Geometry: final body of the model. Coordinates: model frame, mm. Round coordinates to 2 decimals unless told otherwise and drop trailing zeros. Order: outer loops, then holes, each group sorted by start corner. A loop starts at its lowest first (then second) coordinate and runs counter-clockwise, first axis right, second up. Notation, with made-up numbers: M -11,-26 L 8,-26 A21 ccw 8,10 Z; hole C 57,-18 d8. An arc over 180 degrees is marked long. Return JSON: item names as keys, results as strings. Group by question number.
Q1. Ray query, probe 1 along X at (y, z) = (0, -0.6); probe 2 along Y at (x, z) = (1.75, -0.45); probe 3 along Y at (x, z) = (-1, -1.3). Return the intervals inside material, ascending.
Q2. Cut plane C-C on z = -0.8. Output: boundary loops of the cut face in (x, y).
Q3. Cut plane B-B on y = 0. Output: boundary loops of the cut face in (x, z).
Q4. Cut plane A-A on x = 0. Output: boundary loops of the cut face in (y, z).
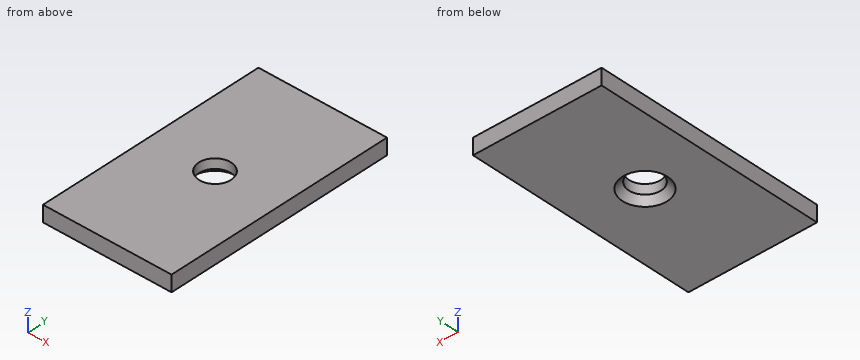
Autodesk Inventor part; units mm, degrees
ref_plane "to_magnet_XY" through (0, 0, 0) normal (0, 0, 1) x (1, 0, 0)
ref_plane "to_magnet_YZ" through (0, 0, 0) normal (1, 0, 0) x (0, 1, 0)
ref_plane "to_magnet_ZX" through (0, 0, 0) normal (0, 1, 0) x (0, 0, 1)
sketch "Sketch_1" plane through (0, 0, 0) normal (0, 0, 1) x (1, 0, 0)
  line L0 (-8, 14.5) -> (-8, -14.5)
  line L1 (-8, -14.5) -> (8, -14.5)
  line L2 (8, -14.5) -> (8, 14.5)
  line L3 (8, 14.5) -> (-8, 14.5)
extrude "Extrusion1" add sketch "Sketch_1" against normal blind 2
sketch "Sketch_2" plane through (0, 0, 0) normal (1, 0, 0) x (0, 1, 0)
  line L0 (0, -2) -> (0, 0)
  line L1 (0, 0) -> (2, 0)
  line L2 (2, 0) -> (2, -1.2)
  line L3 (2, -1.2) -> (2.8, -2)
  line L4 (2.8, -2) -> (0, -2)
  line L5 (0, -2) -> (0, 0)
revolve "Revolution1" cut sketch "Sketch_2" angle 360 about axis through (0, 0, -2) along (0, 0, -1)
ref_plane "to_magnet_XY" through (0, 0, 0) normal (0, 0, 1) x (1, 0, 0)
ref_plane "to_magnet_YZ" through (0, 0, 0) normal (1, 0, 0) x (0, 1, 0)
ref_plane "to_magnet_ZX" through (0, 0, 0) normal (0, 1, 0) x (0, 0, 1)
ref_plane "b1_XY" through (0, -25, -1.2) normal (0, 0, 1) x (1, 0, 0)
ref_plane "b1_YZ" through (0, -25, -1.2) normal (1, 0, 0) x (0, 1, 0)
ref_plane "b1_ZX" through (0, -25, -1.2) normal (0, 1, 0) x (0, 0, 1)
ref_plane "b2_XY" through (0, 25, -1.2) normal (0, 0, 1) x (1, 0, 0)
ref_plane "b2_YZ" through (0, 25, -1.2) normal (1, 0, 0) x (0, 1, 0)
ref_plane "b2_ZX" through (0, 25, -1.2) normal (0, 1, 0) x (0, 0, 1)
ref_plane "bb1_XY" through (0, 0, -1.2) normal (0, 0, 1) x (1, 0, 0)
ref_plane "bb1_YZ" through (0, 0, -1.2) normal (1, 0, 0) x (0, 1, 0)
ref_plane "bb1_ZX" through (0, 0, -1.2) normal (0, 1, 0) x (0, 0, 1)
ref_plane "b2x_XY" through (0, 25, 0) normal (0, 0, 1) x (1, 0, 0)
ref_plane "b2x_YZ" through (0, 25, 0) normal (1, 0, 0) x (0, 1, 0)
ref_plane "b2x_ZX" through (0, 25, 0) normal (0, 1, 0) x (0, 0, 1)
ref_plane "b1x_XY" through (0, -25, 0) normal (0, 0, 1) x (1, 0, 0)
ref_plane "b1x_YZ" through (0, -25, 0) normal (1, 0, 0) x (0, 1, 0)
ref_plane "b1x_ZX" through (0, -25, 0) normal (0, 1, 0) x (0, 0, 1)
properties part number "HMEN5-5-dps"
Result sheet:
{
 "1": {"probe 1": "x = -8 to -2, 2 to 8", "probe 2": "y = -14.5 to -0.97, 0.97 to 14.5", "probe 3": "y = -14.5 to -1.85, 1.85 to 14.5"},
 "2": {"outline": "M -8,-14.5 L 8,-14.5 L 8,14.5 L -8,14.5 Z; hole C 0,0 d4"},
 "3": {"outline": "M -8,-2 L -2.8,-2 L -2,-1.2 L -2,0 L -8,0 Z; M 2,-1.2 L 2.8,-2 L 8,-2 L 8,0 L 2,0 Z"},
 "4": {"outline": "M -14.5,-2 L -2.8,-2 L -2,-1.2 L -2,0 L -14.5,0 Z; M 2,-1.2 L 2.8,-2 L 14.5,-2 L 14.5,0 L 2,0 Z"}
}
